Can you work these out from the model? Positions are in its coordinate system, mm. Coordinates: 2 decimals unless noted, no trailing zeros. Loops run counter-clockwise (first coordinate to the right, second up) from the corner with the lowest first, then second, coordinate; pieces in that order, holes last. Notation, with made-up numbers: (-30.75, -13) -> (-15.75, -13) arc R23 ccw to (-15.75, 20) -> close; hole circle Ø9 at (81.25, -32). An arc over 180 degrees is marked (long way). Use one line per item in the form item = value. Start each with the question number.
(1) Imagine slicing it at A-A (y = -178.92). List the corners of the cut face in (x, z) for me.
(2) Imagine slicing it at C-C (y = -72.5). List the corners of the cut face in (x, z) for me, plus the area to 3 significant figures.
(3) I need wall thicknesses on line 1 (Y direction, x = -175, z = 4); line 2 (X direction, y = -273, z = 5.2); line 3 (Y direction, x = -245, z = 5.6). Which ranges of each line are inside material? Lowest first, please. Write a range as [from, to].
(4) I'm going to push flat-ended pins straight in: pin 1 (3 mm diameter, centred on x = -288.5, z = 2, fed in from +Y); pin 2 (3.5 mm diameter, centred on x = -283, y = -99, fed in from -Z); pin 3 (3 mm diameter, centred on y = -106.5, z = 2, fed in from -X). Where does each tip first touch, or does it pass through?
(5) Imagine slicing it at B-B (x = -238.5). List the corners of the cut face in (y, z) for me, plus the area to 3 significant figures.
(6) Imagine slicing it at D-D (z = 3.9). State how many separate pieces and enclosed holes the cut face has, plus the area to 3 significant figures.
```python
from build123d import *

# Parameters (mm, degrees)
ESQUISSE2_W                            = 330
ESQUISSE2_H                            = 340
BOSS_EXTRU_1_DEPTH                     = 6
ESQUISSE4_W                            = 65
ESQUISSE4_H                            = 6
ESQUISSE4_W_2                          = 40
ESQUISSE4_W_3                          = 6
ESQUISSE4_H_2                          = 68
ENL_V_MAT_ENCOCHE_BORD_DEPTH           = 474.852297662
ESQUISSE5_W                            = 38
ESQUISSE5_H                            = 6
ESQUISSE5_W_2                          = 25
ESQUISSE5_H_2                          = 30
ESQUISSE5_W_3                          = 15
ESQUISSE5_H_3                          = 10
ESQUISSE5_W_4                          = 20
ENL_V_MAT_ENCOCHE_TAGE_ROULETTES_DEPTH = 474.852297662
ESQUISSE6_R                            = 8
ENL_V_MAT_EXTRU_1_DEPTH                = 10
ESQUISSE7_W                            = 165
ESQUISSE7_H                            = 340.861655668
ENL_V_MAT_EXTRU_2_DEPTH                = 474.852297662
ESQUISSE8_R                            = 1.5
ENL_V_MAT_EXTRU_3_DEPTH                = 474.852297662
ESQUISSE9_R                            = 2.995
ESQUISSE9_R_2                          = 3
ENL_V_MAT_EXTRU_4_DEPTH                = 3


with BuildPart() as part:
    # Esquisse2 → Boss.-Extru.1 (new body)
    with BuildSketch(Plane.XY):
        with Locations((-165, -170)):
            Rectangle(ESQUISSE2_W, ESQUISSE2_H)
    extrude(amount=BOSS_EXTRU_1_DEPTH)

    # Esquisse4 → Enlèv. mat encoche bord (cut, through all)
    with BuildSketch(Plane(origin=(0, 0, 0), x_dir=(-1, 0, 0), z_dir=(0, 0, -1))):
        with Locations((297.5, -3)):
            Rectangle(ESQUISSE4_W, ESQUISSE4_H)
        with Locations((205, -3)):
            Rectangle(ESQUISSE4_W_2, ESQUISSE4_H)
        with Locations((125, -3)):
            Rectangle(ESQUISSE4_W_2, ESQUISSE4_H)
        with Locations((32.5, -3)):
            Rectangle(ESQUISSE4_W, ESQUISSE4_H)
        with Locations((327, -102)):
            Rectangle(ESQUISSE4_W_3, ESQUISSE4_H_2)
        with Locations((3, -102)):
            Rectangle(ESQUISSE4_W_3, ESQUISSE4_H_2)
        with Locations((297.5, -337)):
            Rectangle(ESQUISSE4_W, ESQUISSE4_H)
        with Locations((205, -337)):
            Rectangle(ESQUISSE4_W_2, ESQUISSE4_H)
        with Locations((125, -337)):
            Rectangle(ESQUISSE4_W_2, ESQUISSE4_H)
        with Locations((32.5, -337)):
            Rectangle(ESQUISSE4_W, ESQUISSE4_H)
        with Locations((327, -238)):
            Rectangle(ESQUISSE4_W_3, ESQUISSE4_H_2)
        with Locations((3, -238)):
            Rectangle(ESQUISSE4_W_3, ESQUISSE4_H_2)
    extrude(amount=-ENL_V_MAT_ENCOCHE_BORD_DEPTH, mode=Mode.SUBTRACT)

    # Esquisse5 → Enlèv. mat encoche étage + roulettes (cut, through all)
    with BuildSketch(Plane(origin=(0, 0, 0), x_dir=(-1, 0, 0), z_dir=(0, 0, -1))):
        with Locations((251, -273)):
            Rectangle(ESQUISSE5_W, ESQUISSE5_H)
        with Locations((79, -273)):
            Rectangle(ESQUISSE5_W, ESQUISSE5_H)
        with Locations((317.5, -21)):
            Rectangle(ESQUISSE5_W_2, ESQUISSE5_H_2)
        with Locations((7.5, -11)):
            Rectangle(ESQUISSE5_W_3, ESQUISSE5_H_3)
        with Locations((300, -99)):
            Rectangle(ESQUISSE5_W_4, ESQUISSE5_H)
        with Locations((30, -99)):
            Rectangle(ESQUISSE5_W_4, ESQUISSE5_H)
    extrude(amount=-ENL_V_MAT_ENCOCHE_TAGE_ROULETTES_DEPTH, mode=Mode.SUBTRACT)

    # Esquisse6 → Enlèv. mat.-Extru.1 (cut)
    with BuildSketch(Plane.XY.offset(6)):
        with Locations((-21, -178.92)):
            Circle(ESQUISSE6_R)
        with Locations((-309, -178.92)):
            Circle(ESQUISSE6_R)
    extrude(amount=-ENL_V_MAT_EXTRU_1_DEPTH, mode=Mode.SUBTRACT)

    # Esquisse7 → Enlèv. mat.-Extru.2 (cut, through all)
    with BuildSketch(Plane.XY.offset(6)):
        with Locations((-82.5, -170.430827834)):
            Rectangle(ESQUISSE7_W, ESQUISSE7_H)
    extrude(amount=-ENL_V_MAT_EXTRU_2_DEPTH, mode=Mode.SUBTRACT)

    # Esquisse8 → Enlèv. mat.-Extru.3 (cut, through all)
    with BuildSketch(Plane(origin=(0, 0, 0), x_dir=(-1, 0, 0), z_dir=(0, 0, -1))):
        with Locations((175, -337)):
            Circle(ESQUISSE8_R)
        with Locations((232, -337)):
            Circle(ESQUISSE8_R)
        with Locations((258, -337)):
            Circle(ESQUISSE8_R)
        with Locations((327, -331)):
            Circle(ESQUISSE8_R)
        with Locations((327, -303)):
            Circle(ESQUISSE8_R)
        with Locations((327, -279)):
            Circle(ESQUISSE8_R)
        with Locations((277, -273)):
            Circle(ESQUISSE8_R)
        with Locations((225, -273)):
            Circle(ESQUISSE8_R)
        with Locations((327, -197)):
            Circle(ESQUISSE8_R)
        with Locations((327, -170)):
            Circle(ESQUISSE8_R)
        with Locations((327, -143)):
            Circle(ESQUISSE8_R)
        with Locations((327, -61)):
            Circle(ESQUISSE8_R)
        with Locations((327, -43)):
            Circle(ESQUISSE8_R)
        with Locations((258, -3)):
            Circle(ESQUISSE8_R)
        with Locations((232, -3)):
            Circle(ESQUISSE8_R)
        with Locations((175, -3)):
            Circle(ESQUISSE8_R)
        with Locations((317, -99)):
            Circle(ESQUISSE8_R)
        with Locations((283, -99)):
            Circle(ESQUISSE8_R)
    extrude(amount=-ENL_V_MAT_EXTRU_3_DEPTH, mode=Mode.SUBTRACT)

    # Esquisse9 → Enlèv. mat.-Extru.4 (cut)
    with BuildSketch(Plane(origin=(0, 0, 0), x_dir=(-1, 0, 0), z_dir=(0, 0, -1))):
        with Locations((327, -43)):
            Circle(ESQUISSE9_R)
        with Locations((327, -61)):
            Circle(ESQUISSE9_R)
        with Locations((317, -99)):
            Circle(ESQUISSE9_R)
        with Locations((283, -99)):
            Circle(ESQUISSE9_R)
        with Locations((327, -143)):
            Circle(ESQUISSE9_R)
        with Locations((327, -170)):
            Circle(ESQUISSE9_R)
        with Locations((327, -331)):
            Circle(ESQUISSE9_R)
        with Locations((327, -303)):
            Circle(ESQUISSE9_R)
        with Locations((327, -279)):
            Circle(ESQUISSE9_R)
        with Locations((277, -273)):
            Circle(ESQUISSE9_R_2)
        with Locations((225, -273)):
            Circle(ESQUISSE9_R_2)
        with Locations((258, -337)):
            Circle(ESQUISSE9_R)
        with Locations((232, -337)):
            Circle(ESQUISSE9_R)
        with Locations((175, -337)):
            Circle(ESQUISSE9_R)
        with Locations((327, -197)):
            Circle(ESQUISSE9_R)
        with Locations((258, -3)):
            Circle(ESQUISSE9_R)
        with Locations((232, -3)):
            Circle(ESQUISSE9_R)
        with Locations((175, -3)):
            Circle(ESQUISSE9_R)
    extrude(amount=-ENL_V_MAT_EXTRU_4_DEPTH, mode=Mode.SUBTRACT)


solid = part.part
```
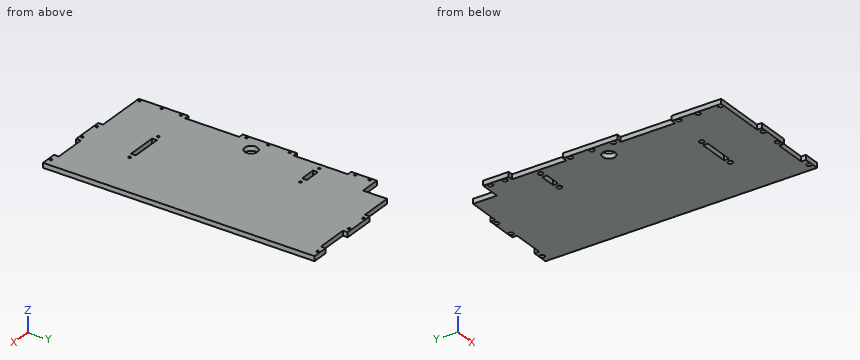
Worked out:
q1.outline = (-330, 0) -> (-317, 0) -> (-317, 6) -> (-330, 6) -> close; (-301, 0) -> (-165, 0) -> (-165, 6) -> (-301, 6) -> close
q2.outline = (-324, 0) -> (-165, 0) -> (-165, 6) -> (-324, 6) -> close
q2.area = 954 mm2
q3.line_1 = [-340, -338.5], [-335.5, -4.5], [-1.5, 0]
q3.line_2 = [-330, -278.5], [-275.5, -270], [-232, -226.5], [-223.5, -165]
q3.line_3 = [-340, -276], [-270, 0]
q4.pin_1 = -6
q4.pin_2 = 3
q4.pin_3 = -324
q5.outline = (-340, 0) -> (-276, 0) -> (-276, 6) -> (-340, 6) -> close; (-270, 0) -> (0, 0) -> (0, 6) -> (-270, 6) -> close
q5.area = 2,000 mm2
q6.separate_pieces = 1
q6.enclosed_holes = 21
q6.area = 52,600 mm2
